Geometry: final body of the model. Coordinates: model frame, mm. Give positions to 0.01 mm unless a question says otherwise; leave off trailing zeros. Write each loop counter-clockwise with the first axis right and the second up, starting at its lowest first coordinate (ties: lowest second). Pieces come first, ordered by that corner, then holes. Notation, with made-up numbers: M -37,1.5 L -27,1.5 A26 cw -27,40.5 Z; hole C 88,45 d8. An arc over 180 degrees is marked long. Use a Markdown table: item, result. Add a question column.
(1) Cut plane D-D (y = 12). Output: boundary loops of the cut face in (x, z), plus the area to 3 significant figures.
(2) Pin query (flat end, axial travel): pin 1 Ø0.9 at (x, z) = (-60.5, 1.5) entering from +Y (3 decimals); pin 2 Ø3 at (y, z) = (17.5, 3.5) entering from -X. Return the tip coordinate at first contact, or that it passes through.
(3) Material intervals for L1, parallel to X at y = 6.35, z = 0.8; L2, parallel to Y at x = -43, z = 1.5 (3 decimals); L3, parallel to X at y = -12.7, z = 0.9, sorted ascending.
(4) Cut plane A-A (x = -109.5). Output: boundary loops of the cut face in (y, z) (3 decimals), plus the area to 3 significant figures.
(5) Cut plane C-C (y = 34.5). Output: boundary loops of the cut face in (x, z), plus the area to 3 significant figures.
(6) Cut plane B-B (y = -12.7). Output: boundary loops of the cut face in (x, z), plus the area to 3 significant figures.
```python
from build123d import *

# Parameters (mm, degrees)
BOSS_EXTRUDE1_OUTLINE_R = 3.556
BOSS_EXTRUDE1_OUTLINE_W = 260.9469
BOSS_EXTRUDE1_OUTLINE_H = 138.1252
BOSS_EXTRUDE1_DEPTH     = 76.2
CUT_EXTRUDE1_DEPTH      = 355.32482824
CUT_EXTRUDE1_DEPTH_BACK = 355.32482824
FILLET1_R               = 2.54
SKETCH7_W               = 260.9469
SKETCH7_H               = 22.1996
CUT_EXTRUDE2_DEPTH      = 347.152897849
FILLET2_R               = 6.35
SKETCH8_W               = 190.775627824
SKETCH8_H               = 235.521960295
CUT_EXTRUDE4_DEPTH      = 347.144751077
SKETCH9_W               = 166.035784577
SKETCH9_H               = 113.418104201
CUT_EXTRUDE5_DEPTH      = 227.747805823


# Read off the part's stored shape, not the designer's step: Boss-Extrude1
with BuildPart() as part:
    # Boss-Extrude1 outline → Boss-Extrude1 (new body)
    with BuildSketch(Plane.XY):
        with BuildLine():
            Line((-286.3596, -22.225), (9.525, -22.225))
            ThreePointArc((9.525, -22.225), (19.05, -12.7), (9.525, -3.175))
            ThreePointArc((9.525, -3.175), (19.05, 6.35), (9.525, 15.875))
            ThreePointArc((9.525, 15.875), (2.789807909, 18.664807909), (0, 25.4))
            Line((0, 25.4), (0, 131.7752))
            ThreePointArc((0, 131.7752), (2.789807909, 138.510392091), (9.525, 141.3002))
            ThreePointArc((9.525, 141.3002), (19.05, 150.8252), (9.525, 160.3502))
            ThreePointArc((9.525, 160.3502), (19.05, 169.8752), (9.525, 179.4002))
            Line((9.525, 179.4002), (-6.35, 179.4002))
            Line((-6.35, 179.4002), (-6.35, 163.5252))
            Line((-6.35, 163.5252), (-7.9502, 163.5252))
            Line((-7.9502, 163.5252), (-7.9502, 160.3502))
            Line((-7.9502, 160.3502), (-268.9098, 160.3502))
            Line((-268.9098, 160.3502), (-268.9098, 163.5252))
            Line((-268.9098, 163.5252), (-270.51, 163.5252))
            Line((-270.51, 163.5252), (-270.51, 179.4002))
            Line((-270.51, 179.4002), (-286.385, 179.4002))
            ThreePointArc((-286.385, 179.4002), (-295.91, 169.8752), (-286.385, 160.3502))
            ThreePointArc((-286.385, 160.3502), (-295.897297883, 150.818850004), (-286.3723, 141.3002))
            ThreePointArc((-286.3723, 141.3002), (-279.637107909, 138.510392091), (-276.8473, 131.7752))
            Line((-276.8473, 131.7752), (-276.8473, 25.4))
            ThreePointArc((-276.8473, 25.4), (-279.637107909, 18.664807909), (-286.3723, 15.875))
            ThreePointArc((-286.3723, 15.875), (-295.8973, 6.35), (-286.3723, -3.175))
            ThreePointArc((-286.3723, -3.175), (-295.884597883, -12.706349996), (-286.3596, -22.225))
        make_face()
        with Locations((-286.3596, -12.7)):
            Circle(BOSS_EXTRUDE1_OUTLINE_R, mode=Mode.SUBTRACT)
        with Locations((-286.3723, 6.35)):
            Circle(BOSS_EXTRUDE1_OUTLINE_R, mode=Mode.SUBTRACT)
        with Locations((9.525, -12.7)):
            Circle(BOSS_EXTRUDE1_OUTLINE_R, mode=Mode.SUBTRACT)
        with Locations((9.525, 6.35)):
            Circle(BOSS_EXTRUDE1_OUTLINE_R, mode=Mode.SUBTRACT)
        with Locations((-286.3723, 150.8252)):
            Circle(BOSS_EXTRUDE1_OUTLINE_R, mode=Mode.SUBTRACT)
        with Locations((-286.385, 169.8752)):
            Circle(BOSS_EXTRUDE1_OUTLINE_R, mode=Mode.SUBTRACT)
        with Locations((-138.42365, 78.5876)):
            Rectangle(BOSS_EXTRUDE1_OUTLINE_W, BOSS_EXTRUDE1_OUTLINE_H, mode=Mode.SUBTRACT)
        with Locations((9.525, 150.8252)):
            Circle(BOSS_EXTRUDE1_OUTLINE_R, mode=Mode.SUBTRACT)
        with Locations((9.525, 169.8752)):
            Circle(BOSS_EXTRUDE1_OUTLINE_R, mode=Mode.SUBTRACT)
    extrude(amount=BOSS_EXTRUDE1_DEPTH)

    # Sketch5 → Cut-Extrude1 (cut, two sides: drawn at the far end of the back side and taken through both)
    with BuildSketch(Plane.ZY.offset(276.8473).offset(-CUT_EXTRUDE1_DEPTH_BACK)):
        Polygon((1.6002, -22.225), (8.641107133, 179.4002), (76.2, 179.4002), (76.2, -22.225), align=None)
    extrude(amount=CUT_EXTRUDE1_DEPTH + CUT_EXTRUDE1_DEPTH_BACK, mode=Mode.SUBTRACT)

    # Fillet1
    fillet1_edges = [part.edges().sort_by_distance(p)[0] for p in [
        (-286.385, 160.3502, 3.987933237),
        (-286.3723, -3.175, 1.132720329),
        (9.525, -3.175, 1.132720329),
        (9.525, 160.3502, 3.987933237),
    ]]
    fillet(fillet1_edges, radius=FILLET1_R)

    # Sketch7 → Cut-Extrude2 (cut, through all)
    with BuildSketch(Plane(origin=(0, 0, 0), x_dir=(-1, 0, 0), z_dir=(0, 0, -1))):
        with Locations((138.42365, -6.35)):
            Rectangle(SKETCH7_W, SKETCH7_H)
    extrude(amount=-CUT_EXTRUDE2_DEPTH, mode=Mode.SUBTRACT)

    # Fillet2
    fillet2_edges = [part.edges().sort_by_distance(p)[0] for p in [
        (-268.8971, 4.7498, 1.271090386),
        (-268.8971, -17.4498, 0.883476829),
        (-7.9502, -17.4498, 0.883476829),
        (-7.9502, 4.7498, 1.271090386),
    ]]
    fillet(fillet2_edges, radius=FILLET2_R)

    # Sketch8 → Cut-Extrude4 (cut, through all)
    with BuildSketch(Plane(origin=(0, -0.082881646, 2.373419811), x_dir=(1, 0, 0), z_dir=(0, -0.03489949670250444, 0.9993908270190958))):
        with Locations((-233.811463912, 74.917246318)):
            Rectangle(SKETCH8_W, SKETCH8_H)
    extrude(amount=-CUT_EXTRUDE4_DEPTH, mode=Mode.SUBTRACT)

    # Sketch9 → Cut-Extrude5 (cut, through all)
    with BuildSketch(Plane(origin=(0, -0.082881646, 2.373419811), x_dir=(1, 0, 0), z_dir=(0, -0.03489949670250444, 0.9993908270190958))):
        with Locations((-55.405757712, 135.427486891)):
            Rectangle(SKETCH9_W, SKETCH9_H)
    extrude(amount=-CUT_EXTRUDE5_DEPTH, mode=Mode.SUBTRACT)


solid = part.part
```
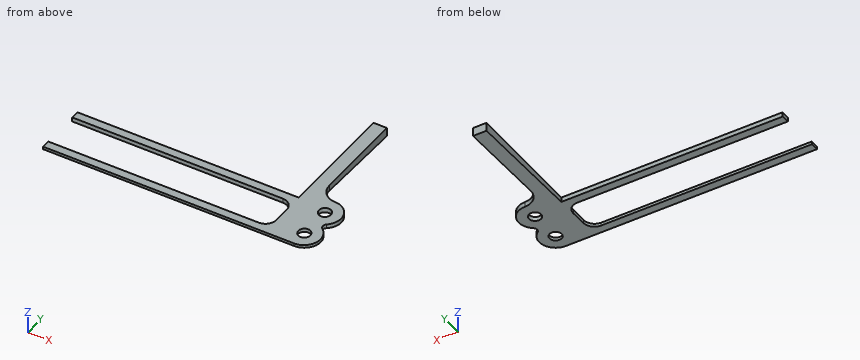
Answer list:
| question | item | result |
|---|---|---|
| 1 | outline | M -7.95,0 L 17.19,0 L 17.19,2.8 L -7.95,2.8 Z |
| 1 | area | 70.3 mm² |
| 2 | pin 1 | y = 9.525 |
| 2 | pin 2 | x = -7.95 |
| 3 | L1 | -138.42 to 5.97, 13.08 to 19.05 |
| 3 | L2 | -22.225 to -17.45, 4.75 to 9.525 |
| 3 | L3 | -8.16 to 5.97, 13.08 to 19.05 |
| 4 | outline | M -22.225,0 L -17.45,0 L -17.45,1.767 L -22.225,1.6 Z; M 4.75,0 L 9.525,0 L 9.525,2.709 L 4.75,2.542 Z |
| 4 | area | 20.6 mm² |
| 5 | outline | M -7.95,0 L 0,0 L 0,3.58 L -7.95,3.58 Z |
| 5 | area | 28.5 mm² |
| 6 | outline | M -8.16,0 L 5.97,0 L 5.97,1.93 L -8.16,1.93 Z; M 13.08,0 L 19.05,0 L 19.05,1.93 L 13.08,1.93 Z |
| 6 | area | 38.8 mm² |
